from build123d import *

# Parameters (mm, degrees)
F0_W      = 40
F0_H      = 20
F1_DEPTH  = 3
F2_W      = 0.05
F2_H      = 6
F3_DEPTH  = 1
F3_FACE_W = 6
F3_FACE_H = 1
F4_DEPTH  = 30
F4_TAPER  = -4


with BuildPart() as f1:
    # F0 (on Top) → F1 (new body)
    with BuildSketch(Plane.XY):
        Rectangle(F0_W, F0_H)
    extrude(amount=F1_DEPTH)

    # F2 (on face) → F3 (join)
    with BuildSketch(Plane.XY.offset(3)):
        with Locations((15.67463018, 0)):
            Rectangle(F2_W, F2_H)
    extrude(amount=F3_DEPTH)

    # F3_face (on face) → F4 (join)
    with BuildSketch(Plane(origin=(15.64963018, 0, 3.5), x_dir=(0, -1, 0), z_dir=(-1, 0, 0))):
        Rectangle(F3_FACE_W, F3_FACE_H)
    extrude(amount=F4_DEPTH, taper=F4_TAPER)


solid = f1.part
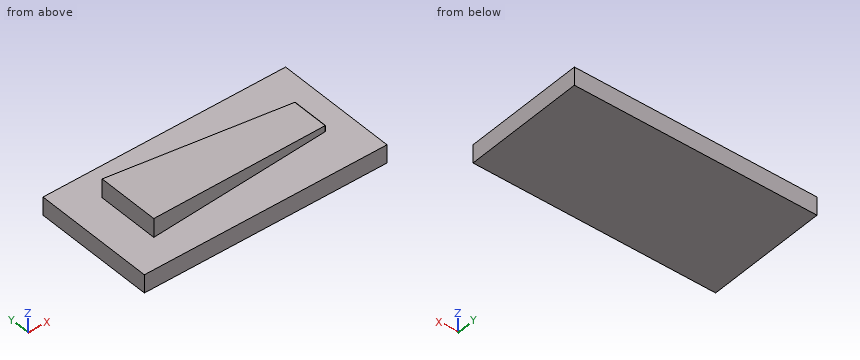
The listing builds one solid part. Answer for the finished solid, in the listing's coordinates (mm). Coordinates: 2 decimals unless noted, no trailing zeros. Loops run counter-clockwise (first coordinate to the right, second up) from the corner with the lowest first, then second, coordinate; pieces in that order, holes last.
1) Find the intervals of material crossed by L1, parallel to Z at x = -9.5, y = 7; L2, parallel to X at y = -2.75, z = 3.5; L3, parallel to Z at x = 0, y = 3.25, in increasing order.
2) Flat-ended cylindrical pins translate along their axes: pin 1 Ø10 at (x, y) = (3, 6.5) entering from +Z; pin 2 Ø0.8 at (y, z) = (-0.5, 3.5) entering from +X; pin 3 Ø10 at (x, y) = (-1.5, -1.5) entering from +Z. Find the tip coordinate at first contact, or state that the pin passes through.
3) Find section A-A on y = 6. Write down the section's boundary in (x, z), then the cut area to 3 significant figures.
Values:
1. L1: z = 0 to 3
1. L2: x = -14.35 to 15.7
1. L3: z = 0 to 5.09
2. pin 1: stops at z = 5.19
2. pin 2: stops at x = 15.7
2. pin 3: stops at z = 5.55
3. outline: (-20, 0) - (20, 0) - (20, 3) - (-20, 3) - close
3. area: 120 mm2
